from build123d import *

# Parameters (mm, degrees)
SKETCH_1_W      = 36
SKETCH_1_H      = 60
EXTRUDE_1_DEPTH = 1210


with BuildPart() as part:
    # Эскиз1 → Вытянуть1 (new body)
    with BuildSketch(Plane.XY):
        Polygon((0, 75), (0, 0), (75, 0), (75, 6), (546, 6), (546, 12), (516, 12), (516, 72), (546, 72), (546, 78), (6, 78), (6, 75), align=None)
        with Locations((495, 42)):
            Rectangle(SKETCH_1_W, SKETCH_1_H, mode=Mode.SUBTRACT)
        with Locations((456, 42)):
            Rectangle(SKETCH_1_W, SKETCH_1_H, mode=Mode.SUBTRACT)
        with Locations((417, 42)):
            Rectangle(SKETCH_1_W, SKETCH_1_H, mode=Mode.SUBTRACT)
        with Locations((378, 42)):
            Rectangle(SKETCH_1_W, SKETCH_1_H, mode=Mode.SUBTRACT)
        with Locations((339, 42)):
            Rectangle(SKETCH_1_W, SKETCH_1_H, mode=Mode.SUBTRACT)
        with Locations((300, 42)):
            Rectangle(SKETCH_1_W, SKETCH_1_H, mode=Mode.SUBTRACT)
        with Locations((261, 42)):
            Rectangle(SKETCH_1_W, SKETCH_1_H, mode=Mode.SUBTRACT)
        with Locations((222, 42)):
            Rectangle(SKETCH_1_W, SKETCH_1_H, mode=Mode.SUBTRACT)
        with Locations((183, 42)):
            Rectangle(SKETCH_1_W, SKETCH_1_H, mode=Mode.SUBTRACT)
        with Locations((144, 42)):
            Rectangle(SKETCH_1_W, SKETCH_1_H, mode=Mode.SUBTRACT)
        with Locations((105, 42)):
            Rectangle(SKETCH_1_W, SKETCH_1_H, mode=Mode.SUBTRACT)
        with Locations((66, 42)):
            Rectangle(SKETCH_1_W, SKETCH_1_H, mode=Mode.SUBTRACT)
        Polygon((45, 12), (16, 12), (16, 6), (6, 6), (6, 72), (45, 72), align=None, mode=Mode.SUBTRACT)
    extrude(amount=-EXTRUDE_1_DEPTH)

    # Зеркальное отражение1: part across face


with BuildPart() as part_1:
    add(part.part)
    add(part.part.mirror(Plane(origin=(546, 9, -605), x_dir=(0, 0, 1), z_dir=(1, 0, 0))))


solid = part_1.part
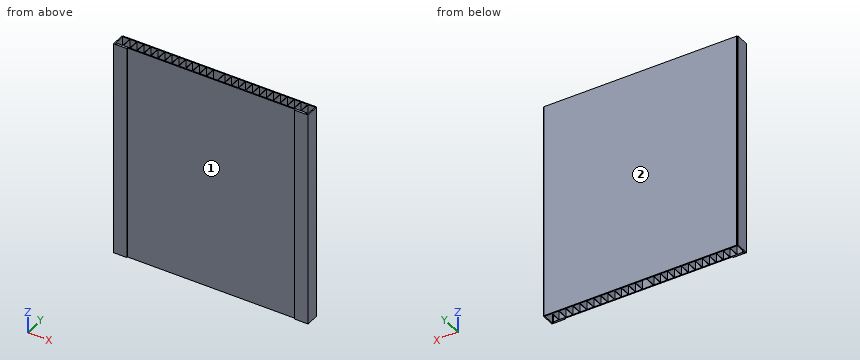
The listing builds one solid part. Answer for the finished solid, in the listing's coordinates (mm). Face numbers are marked on the shaded views. Coordinates: 2 decimals unless noted, no trailing zeros. Loops run counter-clockwise (first coordinate to the right, second up) from the corner with the lowest first, then second, coordinate; pieces in that order, holes last.
1) Determine the mould class of the marked faces 1 and 2 for opening direction X: pulls with the +X half, pulls with the -X half, needs draft (parallel to the pull), parting line crosses it, or undercut.
2) Find section A-A on x = 298. Write down the section's boundary in (y, z), then the cut area to 3 significant figures.
3) Find the intervals of material crossed by L1, parallel to Y at x = 313.5, z = -181.5; L2, parallel to X at y = 6.5, z = -1066; L3, parallel to Y at x = 57, z = -755.5, in increasing order.
4) Find section B-B on y = 41.5. Give the number of separate pieces and of enclosed holes in the cut face, then the cut area to 3 significant figures.
5) Flat-ended cylindrical pins translate along their axes: pin 1 Ø18 at (x, z) = (386, -599.5) entering from -Y; pin 2 Ø12 at (x, y) = (663.5, 21) entering from -Z. Find the tip coordinate at first contact, or state that the pin passes through.
Values:
1. face 1: undercut
1. face 2: needs draft
2. outline: (6, -1210) - (12, -1210) - (12, 0) - (6, 0) - close; (72, -1210) - (78, -1210) - (78, 0) - (72, 0) - close
2. area: 14,500 mm2
3. L1: y = 6 to 12, 72 to 78
3. L2: x = 0 to 6, 16 to 1076, 1086 to 1092
3. L3: y = 0 to 12, 72 to 78
4. separate pieces: 28
4. enclosed holes: 0
4. area: 109,000 mm2
5. pin 1: stops at y = 6
5. pin 2: passes through
